from build123d import *

# Parameters (mm, degrees)
BOSS_EXTRUDE1_DEPTH            = 6.35
F_6_CLEARANCE_HOLE1_AT_2_COUNT = 2
F_6_CLEARANCE_HOLE1_AT_2_PITCH = 12.7
F_6_CLEARANCE_HOLE2_AT_2_COUNT = 2
F_6_CLEARANCE_HOLE2_AT_2_PITCH = 12.7


with BuildPart() as part:
    # Sketch1 → Boss-Extrude1 (new, symmetric)
    with BuildSketch(Plane(origin=(0, 0, 0), x_dir=(0, 0, -1), z_dir=(1, 0, 0))):
        with BuildLine():
            Line((0, 3.175), (0, 38.1))
            Line((0, 38.1), (1.524, 38.1))
            Line((1.524, 38.1), (1.524, 3.175))
            ThreePointArc((1.524, 3.175), (2.007566704, 2.007566704), (3.175, 1.524))
            Line((3.175, 1.524), (38.1, 1.524))
            Line((38.1, 1.524), (38.1, 0))
            Line((38.1, 0), (3.175, 0))
            ThreePointArc((3.175, 0), (0.92993597, 0.92993597), (0, 3.175))
        make_face()
    extrude(amount=BOSS_EXTRUDE1_DEPTH, both=True)

    # Sketch3 → #6 Clearance Hole1 (revolve, cut)
    with BuildSketch(Plane(origin=(0, 1.524, -25.4), x_dir=(0, 0, 1), z_dir=(1, 0, 0))):
        Polygon((0, 0), (0, 1.524), (2.15265, 1.524), (2.15265, 1.02235), (3.175, 0), align=None)
    f_6_clearance_hole1 = revolve(axis=Axis((0, 7.874, -25.4), (0, -1, 0)), mode=Mode.SUBTRACT)

    # #6 Clearance Hole1 at 2: #6 Clearance Hole1 ×2
    with Locations(*[(0, 0, i * F_6_CLEARANCE_HOLE1_AT_2_PITCH) for i in range(1, F_6_CLEARANCE_HOLE1_AT_2_COUNT)]):
        add(f_6_clearance_hole1, mode=Mode.SUBTRACT)

    # Sketch6 → #6 Clearance Hole2 (revolve, cut)
    with BuildSketch(Plane(origin=(0, 12.7, -1.524), x_dir=(0, 1, 0), z_dir=(1, 0, 0))):
        Polygon((0, 0), (0, 1.524), (2.15265, 1.524), (2.15265, 1.02235), (3.175, 0), align=None)
    f_6_clearance_hole2 = revolve(axis=Axis((0, 12.7, -7.874), (0, 0, 1)), mode=Mode.SUBTRACT)

    # #6 Clearance Hole2 at 2: #6 Clearance Hole2 ×2
    with Locations(*[(0, i * F_6_CLEARANCE_HOLE2_AT_2_PITCH, 0) for i in range(1, F_6_CLEARANCE_HOLE2_AT_2_COUNT)]):
        add(f_6_clearance_hole2, mode=Mode.SUBTRACT)


solid = part.part
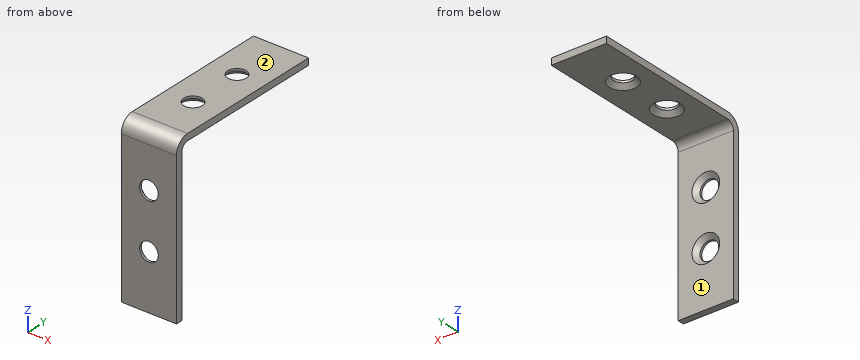
Read the model definition and answer for the solid it produces. Units are mm, in the model's axes. Face numbers are marked on the shaded views. A direction names the side the tool comes from. Give positions to 0.01 mm unless a question says otherwise; leave off trailing zeros. Write each loop counter-clockwise with the first axis right and the second up, starting at its lowest first coordinate (ties: lowest second). Pieces come first, ordered by that corner, then holes. Notation, with made-up numbers: (57, -37) -> (62, -37) arc R27 cw to (62, -1) -> close; hole circle Ø9 at (29.25, -6). An arc over 180 degrees is marked (long way). Answer as a JSON object with one key per item and string values. Group by question number.
1) Each of these flat-tipped pins is pushed along its axis until it touches: P1, Ø2.5, axis at x = 0, z = -25.4, coming from the -Y side; P2, Ø1.5, axis at x = -4.5, y = 18, coming from the -Z side; P3, Ø2, axis at x = 2.5, z = -32.5, coming from the +Y side. Where does it stop, or does it pass through?
2) A tool of negligible diameter and unlimited length cuts with its end or side. For the marked faces 1 and 2, from which of +Z, -Z, +X, -X, +Y, -Y can it reach the whole face along a straight path? Write none if from no direction.
3) Find section B-B (x = 0). Count the separate pieces of the cut face and the enclosed holes in it, and give its area (3 significant figures).
4) Find section D-D (x = 4.75). Write down the section's boundary in (y, z) (3 decimals), and give its area (3 significant figures).
5) Find section C-C (z = -12.7). Write down the section's boundary in (x, y) (3 decimals), and give its area (3 significant figures).
6) Consider L1, parallel to X at y = 0.35, z = -25.4; L2, parallel to Z at x = 0, y = 0.35; L3, parallel to Z at x = 0, y = 0.25. Determine where each line is inside the solid, lowest interval first. Write a range as from..to.
7) Find section A-A (y = 25.4). Write down the section's boundary in (x, z) (3 decimals), and give its area (3 significant figures).
Values follow:
{
 "1": {"P1": "passes through", "P2": "stops at z = -1.52", "P3": "stops at y = 1.52"},
 "2": {"face 1": "-Z, +X, -X, +Y", "face 2": "+Z, +X, -X, +Y, -Y"},
 "3": {"separate pieces": "5", "enclosed holes": "0", "area": "81.8 mm2"},
 "4": {"outline": "(0, -38.1) -> (1.524, -38.1) -> (1.524, -3.175) arc R1.651 cw to (3.175, -1.524) -> (38.1, -1.524) -> (38.1, 0) -> (3.175, 0) arc R3.175 ccw to (0, -3.175) -> close", "area": "112 mm2"},
 "5": {"outline": "(-6.35, 0) -> (-2.153, 0) -> (-2.153, 0.502) -> (-3.175, 1.524) -> (-6.35, 1.524) -> close; (2.153, 0) -> (6.35, 0) -> (6.35, 1.524) -> (3.175, 1.524) -> (2.153, 0.502) -> close", "area": "11.7 mm2"},
 "6": {"L1": "x = -6.35..-2.15, 2.15..6.35", "L2": "z = -38.1..-27.55, -23.25..-14.85, -10.55..-1.73", "L3": "z = -38.1..-27.55, -23.25..-14.85, -10.55..-1.94"},
 "7": {"outline": "(-6.35, -1.524) -> (-3.175, -1.524) -> (-2.153, -0.502) -> (-2.153, 0) -> (-6.35, 0) -> close; (2.153, -0.502) -> (3.175, -1.524) -> (6.35, -1.524) -> (6.35, 0) -> (2.153, 0) -> close", "area": "11.7 mm2"}
}
